For this review, take the finished solid that the model builds, in its own axes (mm). Face numbers are marked on the shaded views. A direction names the side the tool comes from. Coordinates: 2 decimals unless noted, no trailing zeros. Write each loop counter-clockwise with the first axis right and the second up, starting at its lowest first coordinate (ties: lowest second). Pieces come first, ordered by that corner, then holes. Notation, with made-up numbers: M 61.5,35 L 119.5,35 A6 cw 119.5,43 Z; hole C -21.5,0.25 d5. An arc over 180 degrees is marked long. One line per question, with ' | ' between items.
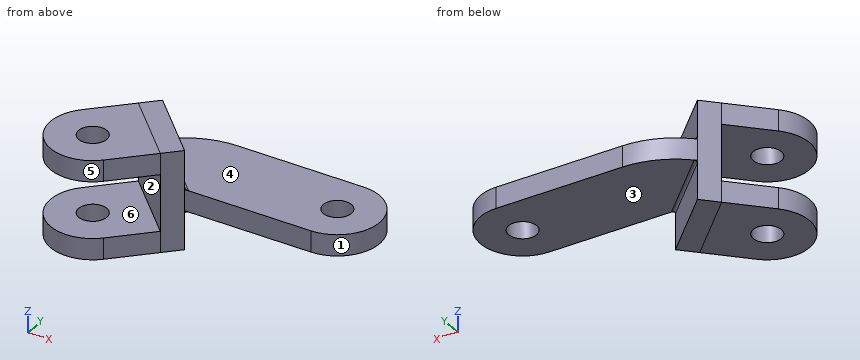
Autodesk Inventor part; units mm, degrees
ref_plane "YZ Plane" through (0, 0, 0) normal (1, 0, 0) x (0, 1, 0)
ref_plane "XZ Plane" through (0, 0, 0) normal (0, 1, 0) x (-1, 0, 0)
ref_plane "XY Plane" through (0, 0, 0) normal (0, 0, 1) x (1, 0, 0)
sketch "Sketch1" plane through (0, 0, 0) normal (0, 0, 1) x (1, 0, 0)
  line L0 (0, -3.3292) -> (0, 5.126)
  line L1 (-4.3113, 0) -> (11.0184, 0)
  line L2 (-1.0607, 1.0607) -> (0.7071, 2.8284)
  arc A0 (2.8284, 3.7071) -> (0.7071, 2.8284) centre (2.8284, 0.7071) ccw
  line L3 (2.8284, 3.7071) -> (7.3284, 3.7071)
  arc A1 (7.3284, 0.7071) -> (7.3284, 3.7071) centre (7.3284, 2.2071) ccw
  line L4 (7.3284, 0.7071) -> (2.8284, 0.7071)
  line L5 (2.8284, 0.7071) -> (1.0607, -1.0607)
  arc A2 (-1.0607, 1.0607) -> (1.0607, -1.0607) centre (0, 0) ccw
  circle A3 centre (0, 0) radius 0.5
  circle A4 centre (7.3284, 2.2071) radius 0.5
  line L6 (2.8284, 0.7071) -> (0.7071, 2.8284)
  line L7 (2.2981, 0.1768) -> (0.1768, 2.2981)
  line L8 (2.2981, 0.1768) -> (2.2981, 0.1768)
  dimension "d0" = 4.5
  dimension "d1" = 45
  dimension "d2" = 1
  dimension "d3" = 1
  dimension "d5" = 2.5
  dimension "d6" = 1.5
  dimension "d8" = 2.5
  dimension "d9" = 1.5
extrude "Extrusion1" add sketch "Sketch1" along normal mid plane 0.75 contours L6 A0 L3 A1 L4
extrude "Extrusion2" add sketch "Sketch1" along normal mid plane 3.5 contours L7 L2 L6 L5
extrude "Extrusion3" add sketch "Sketch1" along normal mid plane 3.5 contours A2 L1 A3 L0 | L0 A3 L1 L5 A2 | A2 L2 L0 A3 L1 | A3 L0 L2 L7 L5 L1
extrude "Extrusion4" cut sketch "Sketch1" along normal mid plane 2 contours A2 L1 A3 L0 | L0 A3 L1 L5 A2 | A2 L2 L0 A3 L1 | A3 L0 L2 L7 L5 L1
fillet "Fillet1" radius 0.1 2 edges at (1.7678, 1.7678, 0.375) (1.7678, 1.7678, -0.375)
properties part number "7c"
1. Take a section at D-D on y = -0.7. State the section outline as (x, z) points, plus the area to 3 significant figures.
Computed values:
outline: M -1.33,-1.75 L 1.42,-1.75 L 1.42,-1 L -1.33,-1 Z; M -1.33,1 L 1.42,1 L 1.42,1.75 L -1.33,1.75 Z | area: 4.12 mm2
2. Take a section at A-A on y = 0. State the section outline as (x, z) points.
Computed values:
outline: M -1.5,-1.75 L -0.5,-1.75 L -0.5,-1 L -1.5,-1 Z; M -1.5,1 L -0.5,1 L -0.5,1.75 L -1.5,1.75 Z; M 0.5,-1.75 L 2.12,-1.75 L 2.12,-1 L 0.5,-1 Z; M 0.5,1 L 2.12,1 L 2.12,1.75 L 0.5,1.75 Z
3. For line 1 along Z through (x, y) = (1, 0.85); line 2 along X through (y, z) = (0, 1.3), list the stretches that pass through material, from the lowest coordinate up.
Computed values:
line 1: z = -1.75 to -1, 1 to 1.75 | line 2: x = -1.5 to -0.5, 0.5 to 2.12
4. Take a section at B-B on x = 7. State the section outline as (y, z) points (3 decimals), plus the area to 3 significant figures.
Computed values:
outline: M 0.707,-0.375 L 1.83,-0.375 L 1.83,0.375 L 0.707,0.375 Z; M 2.584,-0.375 L 3.707,-0.375 L 3.707,0.375 L 2.584,0.375 Z | area: 1.68 mm2
5. Clearance check with a flat-ended pin moving along its axis: P1, Ø1.5, axis at x = 3, y = 2.5, coming from the -Z side (3 decimals). State where the tip first meets the part, or that it passes through.
Computed values:
P1: stops at z = -0.375
6. Draft analysis for pull direction Z (two halves, no side actions). For the marked faces 1, 2, 3 and 4, state which applies: pulls with the +Z half, pulls with the -Z half, needs draft (parallel to the pull), parting line crosses it, or undercut.
Computed values:
face 1: needs draft | face 2: undercut | face 3: pulls with the -Z half | face 4: pulls with the +Z half
7. Machinability: for the marked faces 5 and 6, which of the approach directions +Z, -Z, +X, -X, +Y, -Y give a long, thin tool a straight path to every point of the face, cutting with its end or side? Answer none if there is none.
Computed values:
face 5: +Z, -Z | face 6: -X, -Y
